```python
from build123d import *

# Parameters (mm, degrees)
EXTRUDE_THIN1_START          = -7.9375
EXTRUDE_THIN1_DEPTH          = 15.875
SKETCH4_R                    = 2.3495
EXTRUDE3_DEPTH               = 69.543095394
SKETCH7_R                    = 3.5433
CUT_EXTRUDE1_DEPTH           = 72.040836075
CUT_EXTRUDE1_DRAFT           = -49
CUT_EXTRUDE1_PROFILE_2_DEPTH = 72.040836075
CUT_EXTRUDE1_PROFILE_2_DRAFT = -49
CIRPATTERN1_COUNT            = 2
CIRPATTERN1_COPY_1_SKETCH_R  = 3.5433
CIRPATTERN1_COPY_1_DEPTH     = 72.040836075
CIRPATTERN1_COPY_1_DRAFT     = -49
CIRPATTERN1_COPY_2_SKETCH_R  = 3.5433
CIRPATTERN1_COPY_2_DEPTH     = 72.040836075
CIRPATTERN1_COPY_2_DRAFT     = -49
CIRPATTERN1_COPY_3_SKETCH_R  = 3.5433
CIRPATTERN1_COPY_3_DEPTH     = 72.040836075
CIRPATTERN1_COPY_3_DRAFT     = -49


# Read off the part's stored shape, not the designer's step: Extrude-Thin1
with BuildPart() as part:
    # Extrude-Thin1 outline → Extrude-Thin1 (new body)
    with BuildSketch(Plane(origin=(0, 0, 0), x_dir=(1, 0, 0), z_dir=(0, 1, 0)).offset(EXTRUDE_THIN1_START)):
        with BuildLine():
            Line((2.667, -1.778), (50.8, -1.778))
            Line((50.8, -1.778), (50.8, 0))
            Line((50.8, 0), (2.667, 0))
            ThreePointArc((2.667, 0), (0.781146215, -0.781146215), (0, -2.667))
            Line((0, -2.667), (0, -50.8))
            Line((0, -50.8), (1.778, -50.8))
            Line((1.778, -50.8), (1.778, -2.667))
            ThreePointArc((1.778, -2.667), (2.038382072, -2.038382072), (2.667, -1.778))
        make_face()
    extrude(amount=EXTRUDE_THIN1_DEPTH)

    # Sketch4 → Extrude3 (cut, through all)
    with BuildSketch(Plane(origin=(3.556, 0, 1.778), x_dir=(1, 0, 0), z_dir=(0, 0, 1))):
        with Locations((38.354, 0)):
            Circle(SKETCH4_R)
        with Locations((15.24, 0)):
            Circle(SKETCH4_R)
    extrude3 = extrude(amount=-EXTRUDE3_DEPTH, mode=Mode.SUBTRACT)


with BuildPart() as cut_extrude1_tool:
    # Sketch7 → Cut-Extrude1 (with draft: the straight prism first)
    with BuildSketch(Plane.XY.offset(1.778)):
        with Locations((41.91, 0)):
            Circle(SKETCH7_R)
    extrude(amount=-CUT_EXTRUDE1_DEPTH)
    # Cut-Extrude1: the draft: its side faces are tilted about the plane it starts from
    cut_extrude1_sides = [cut_extrude1_tool.faces().sort_by_distance(p)[0] for p in [
        (38.3667, 0, -34.242418038),
    ]]
    draft(cut_extrude1_sides, Plane.XY.offset(1.778), CUT_EXTRUDE1_DRAFT)


with BuildPart() as part_1:
    add(part.part)

    # Cut-Extrude1: cut by cut_extrude1_tool
    add(cut_extrude1_tool.part, mode=Mode.SUBTRACT)


with BuildPart() as cut_extrude1_profile_2_tool:
    # Sketch7 → Cut-Extrude1 profile 2 (with draft: the straight prism first)
    with BuildSketch(Plane.XY.offset(1.778)):
        with Locations((18.796, 0)):
            Circle(SKETCH7_R)
    extrude(amount=-CUT_EXTRUDE1_PROFILE_2_DEPTH)
    # Cut-Extrude1 profile 2: the draft: its side faces are tilted about the plane it starts from
    cut_extrude1_profile_2_sides = [cut_extrude1_profile_2_tool.faces().sort_by_distance(p)[0] for p in [
        (15.2527, 0, -34.242418038),
    ]]
    draft(cut_extrude1_profile_2_sides, Plane.XY.offset(1.778), CUT_EXTRUDE1_PROFILE_2_DRAFT)


with BuildPart() as part_2:
    add(part_1.part)

    # Cut-Extrude1 profile 2: cut by cut_extrude1_profile_2_tool
    add(cut_extrude1_profile_2_tool.part, mode=Mode.SUBTRACT)

    # CirPattern1: Extrude3 ×2 about axis
    cirpattern1_axis = Axis((0, 0, 0), (0.7071067811865464, 0, 0.7071067811865487))
    for i in range(1, CIRPATTERN1_COUNT):
        add(extrude3.rotate(cirpattern1_axis, i * 360 / CIRPATTERN1_COUNT), mode=Mode.SUBTRACT)


with BuildPart() as cirpattern1_copy_1_tool:
    # CirPattern1 copy 1 sketch → CirPattern1 copy 1 (with draft: the straight prism first)
    with BuildSketch(Plane(origin=(1.778, 0, 0), x_dir=(0, 0, 1), z_dir=(1, 0, 0))):
        with Locations((41.91, 0)):
            Circle(CIRPATTERN1_COPY_1_SKETCH_R)
    extrude(amount=-CIRPATTERN1_COPY_1_DEPTH)
    # CirPattern1 copy 1: the draft: its side faces are tilted about the plane it starts from
    cirpattern1_copy_1_sides = [cirpattern1_copy_1_tool.faces().sort_by_distance(p)[0] for p in [
        (-34.242418038, 0, 38.3667),
    ]]
    draft(cirpattern1_copy_1_sides, Plane(origin=(1.778, 0, 0), x_dir=(0, 0, 1), z_dir=(1, 0, 0)), CIRPATTERN1_COPY_1_DRAFT)


with BuildPart() as part_3:
    add(part_2.part)

    # CirPattern1 copy 1: cut by cirpattern1_copy_1_tool
    add(cirpattern1_copy_1_tool.part, mode=Mode.SUBTRACT)


with BuildPart() as cirpattern1_copy_2_tool:
    # CirPattern1 copy 2 sketch → CirPattern1 copy 2 (with draft: the straight prism first)
    with BuildSketch(Plane(origin=(1.778, 0, 0), x_dir=(0, 0, 1), z_dir=(1, 0, 0))):
        with Locations((18.796, 0)):
            Circle(CIRPATTERN1_COPY_2_SKETCH_R)
    extrude(amount=-CIRPATTERN1_COPY_2_DEPTH)
    # CirPattern1 copy 2: the draft: its side faces are tilted about the plane it starts from
    cirpattern1_copy_2_sides = [cirpattern1_copy_2_tool.faces().sort_by_distance(p)[0] for p in [
        (-34.242418038, 0, 15.2527),
    ]]
    draft(cirpattern1_copy_2_sides, Plane(origin=(1.778, 0, 0), x_dir=(0, 0, 1), z_dir=(1, 0, 0)), CIRPATTERN1_COPY_2_DRAFT)


with BuildPart() as part_4:
    add(part_3.part)

    # CirPattern1 copy 2: cut by cirpattern1_copy_2_tool
    add(cirpattern1_copy_2_tool.part, mode=Mode.SUBTRACT)


with BuildPart() as cirpattern1_copy_3_tool:
    # CirPattern1 copy 3 sketch → CirPattern1 copy 3 (with draft: the straight prism first)
    with BuildSketch(Plane(origin=(1.778, 0, 0), x_dir=(0, 0, 1), z_dir=(1, 0, 0))):
        with Locations((18.796, 0)):
            Circle(CIRPATTERN1_COPY_3_SKETCH_R)
    extrude(amount=-CIRPATTERN1_COPY_3_DEPTH)
    # CirPattern1 copy 3: the draft: its side faces are tilted about the plane it starts from
    cirpattern1_copy_3_sides = [cirpattern1_copy_3_tool.faces().sort_by_distance(p)[0] for p in [
        (-34.242418038, 0, 15.2527),
    ]]
    draft(cirpattern1_copy_3_sides, Plane(origin=(1.778, 0, 0), x_dir=(0, 0, 1), z_dir=(1, 0, 0)), CIRPATTERN1_COPY_3_DRAFT)


with BuildPart() as part_5:
    add(part_4.part)

    # CirPattern1 copy 3: cut by cirpattern1_copy_3_tool
    add(cirpattern1_copy_3_tool.part, mode=Mode.SUBTRACT)


solid = part_5.part
```
Read the model definition and answer for the solid it produces. Units are mm, in the model's axes. A direction names the side the tool comes from. Coordinates: 2 decimals unless noted, no trailing zeros. Write each loop counter-clockwise with the first axis right and the second up, starting at its lowest first coordinate (ties: lowest second). Pieces come first, ordered by that corner, then holes. Notation, with made-up numbers: (31.5, -39) -> (43.5, -39) arc R37 cw to (43.5, 0) -> close; hole circle Ø1 at (0.5, -33.5). An arc over 180 degrees is marked (long way). Return JSON: item names as keys, results as strings.
1. Find the intervals of material crossed by line 1 along Y through (x, z) = (0.6, 41.91); line 2 along X through (y, z) = (-2, 25), in increasing order. Write a range as from..to.
Found:
{"line 1": "-7.94..-2.35, 2.35..7.94", "line 2": "0..1.78"}
2. A tool of negligible diameter and unlimited length cuts with its end or side. For faces 4 (the face through (0.8, -0.11, 0.76)), 5 (the face through (1.778, 0, 27)), from which of +Z, -Z, +X, -X, +Y, -Y can it reach the whole face along a straight path? Write none if from no direction.
Found:
{"face 4": "-Z, -X, +Y, -Y", "face 5": "+Z, +X, +Y, -Y"}
3. A cutting plane is placed at D-D (x = 24). Determine the outline of the cut face in (y, z), and give its area (3 significant figures).
Found:
{"outline": "(-7.94, 0) -> (7.94, 0) -> (7.94, 1.78) -> (-7.94, 1.78) -> close", "area": "28.2 mm2"}
4. Each of these flat-tipped pins is pushed along its axis until it touches: P1, Ø8, axis at x = 24.5, y = -1.5, coming from the +Z side; P2, Ø8, axis at y = -1.5, z = 33, coming from the +X side; P3, Ø5.5, axis at x = 18.796, y = 0, coming from the +Z side. Where does it stop, or does it pass through?
Found:
{"P1": "z = 1.78", "P2": "x = 1.78", "P3": "z = 1.09"}
5. Determine the mould class of faces 1 (the face through (44.15, 0.71, 0.38)), 2 (the face through (14, 7.938, 1)), 3 (the face through (50.8, 0, 1)) for opening direction Y: pulls with the +Y half, pulls with the -Y half, needs draft (parallel to the pull), parting line crosses it, or undercut.
Found:
{"face 1": "undercut", "face 2": "pulls with the +Y half", "face 3": "needs draft"}
6. A cutting plane is placed at B-B (y = 0). Give the number of separate pieces and of enclosed holes in the cut face, and give its area (3 significant figures).
Found:
{"separate pieces": "5", "enclosed holes": "0", "area": "138 mm2"}
7. A cutting plane is placed at C-C (z = 41.91). Determine the outline of the cut face in (x, y), and give its area (3 significant figures).
Found:
{"outline": "(0, -7.94) -> (1.78, -7.94) -> (1.78, -3.54) -> (0.74, -2.35) -> (0, -2.35) -> close; (0, 2.35) -> (0.74, 2.35) -> (1.78, 3.54) -> (1.78, 7.94) -> (0, 7.94) -> close", "area": "18.6 mm2"}
8. A cutting plane is placed at A-A (x = 41.91). Determine the outline of the cut face in (y, z), and give its area (3 significant figures).
Found:
{"outline": "(-7.94, 0) -> (-2.35, 0) -> (-2.35, 0.74) -> (-3.54, 1.78) -> (-7.94, 1.78) -> close; (2.35, 0) -> (7.94, 0) -> (7.94, 1.78) -> (3.54, 1.78) -> (2.35, 0.74) -> close", "area": "18.6 mm2"}
